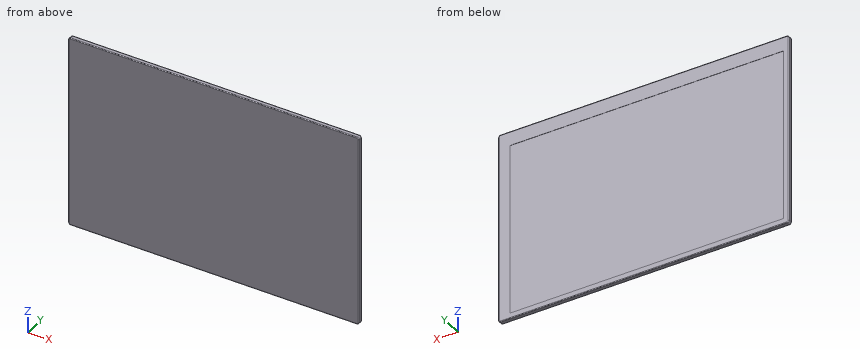
Autodesk Inventor part; units mm, degrees
ref_plane "YZ Plane" through (0, 0, 0) normal (1, 0, 0) x (0, 1, 0)
ref_plane "XZ Plane" through (0, 0, 0) normal (0, 1, 0) x (-1, 0, 0)
ref_plane "XY Plane" through (0, 0, 0) normal (0, 0, 1) x (1, 0, 0)
sketch "Sketch1" plane through (0, 0, 0) normal (0, 1, 0) x (-1, 0, 0)
  line L0 (0, 0) -> (-161.5, 0)
  line L1 (-161.5, 0) -> (-161.5, -107)
  line L2 (-161.5, -107) -> (0, -107)
  line L3 (0, -107) -> (0, 0)
  dimension "d0" = 161.5
  dimension "d1" = 107
extrude "Extrusion1" add sketch "Sketch1" along normal blind 2.5
sketch "Sketch2" plane through (0, 2.5, 0) normal (0, 1, 0) x (1, 0, 0)
  line L0 (161.5, 107) -> (0, 107)
  line L1 (0, 107) -> (0, 0)
  line L2 (3, 104) -> (155, 104)
  line L3 (155, 104) -> (155, 8)
  line L4 (155, 8) -> (3, 8)
  line L5 (3, 8) -> (3, 104)
  dimension "d4" = 3
  dimension "d5" = 3
  dimension "d6" = 152
  dimension "d7" = 96
extrude "Extrusion2" cut sketch "Sketch2" against normal blind 0.1
fillet "Fillet1" radius 0.4 8 edges at (0, 2.5, -53.5) (80.75, 2.5, -107) (80.75, 2.5, 0) (161.5, 2.5, -53.5) (80.75, 0, 0) (0, 0, -53.5) (80.75, 0, -107) (161.5, 0, -53.5)
fillet "Fillet2" radius 1.2 12 edges at (161.3828, 2.3828, -0.1172) (161.3828, 0.1172, -0.1172) (161.5, 1.25, 0) (0.1172, 2.3828, -0.1172) (0.1172, 0.1172, -0.1172) (0, 1.25, 0) (0.1172, 2.3828, -106.8828) (0.1172, 0.1172, -106.8828) (0, 1.25, -107) (161.3828, 2.3828, -106.8828) (161.3828, 0.1172, -106.8828) (161.5, 1.25, -107)
properties part number "main_lcd_panel"
Can you work these out from the model? Positions are in its coordinate system, mm. Coordinates: 2 decimals unless noted, no trailing zeros. Write each loop counter-clockwise with the first axis right and the second up, starting at its lowest first coordinate (ties: lowest second). Pieces come first, ordered by that corner, then holes. Notation, with made-up numbers: (61.25, 38.25) -> (102.25, 38.25) arc R9 ccw to (102.25, 54.25) -> close; hole circle Ø2 at (-18, 26.5). An arc over 180 degrees is marked (long way). Write item = value, one per line.
(1) Imagine slicing it at B-B (x = 111.5). Please give me the cut outline in (y, z).
Verdict:
outline = (0, -106.6) arc R0.4 ccw to (0.4, -107) -> (2.1, -107) arc R0.4 ccw to (2.5, -106.6) -> (2.5, -104) -> (2.4, -104) -> (2.4, -8) -> (2.5, -8) -> (2.5, -0.4) arc R0.4 ccw to (2.1, 0) -> (0.4, 0) arc R0.4 ccw to (0, -0.4) -> close
(2) If I drill on probe 1 along Y at (x, z) = (151, -34); probe 2 along X at (y, z) = (0.35, -89); probe 3 along Z at (x, y) = (45.5, 2.2), over which ranges is the centre line in solid material (lowest first)?
Verdict:
probe_1 = 0 to 2.4
probe_2 = 0 to 161.5
probe_3 = -106.99 to -0.01
(3) Imagine slicing it at A-A (z = -67.5). Please give me the cut outline in (x, y), and give its area (3 significant figures).
Verdict:
outline = (0, 0.4) arc R0.4 ccw to (0.4, 0) -> (161.1, 0) arc R0.4 ccw to (161.5, 0.4) -> (161.5, 2.1) arc R0.4 ccw to (161.1, 2.5) -> (155, 2.5) -> (155, 2.4) -> (3, 2.4) -> (3, 2.5) -> (0.4, 2.5) arc R0.4 ccw to (0, 2.1) -> close
area = 388 mm^2
